```python
from build123d import *

# Parameters (mm, degrees)
SKETCH1_W           = 180
SKETCH1_H           = 87
BOSS_EXTRUDE1_DEPTH = 2
SKETCH6_W           = 2
SKETCH6_H           = 87
BOSS_EXTRUDE5_DEPTH = 5
SKETCH7_R           = 37.5
CUT_EXTRUDE2_DEPTH  = 5
SKETCH8_W           = 87
SKETCH8_H           = 87
SKETCH8_W_2         = 81
SKETCH8_H_2         = 81
BOSS_EXTRUDE6_DEPTH = 5
SKETCH9_W           = 150
SKETCH9_H           = 3
BOSS_EXTRUDE7_DEPTH = 5
SKETCH10_W          = 2
SKETCH10_H          = 87
CUT_EXTRUDE3_DEPTH  = 5
SKETCH11_W          = 2
SKETCH11_H          = 81
BOSS_EXTRUDE8_DEPTH = 5
SKETCH12_R          = 7.5
CUT_EXTRUDE4_DEPTH  = 5


with BuildPart() as part:
    # Sketch1 → Boss-Extrude1 (new body)
    with BuildSketch(Plane(origin=(0, 0, 0), x_dir=(1, 0, 0), z_dir=(0, 1, 0))):
        with Locations((31.597011279, 2.798063398)):
            Rectangle(SKETCH1_W, SKETCH1_H)
    extrude(amount=BOSS_EXTRUDE1_DEPTH)

    # Sketch6 → Boss-Extrude5 (add)
    with BuildSketch(Plane(origin=(0, 0, 0), x_dir=(-1, 0, 0), z_dir=(0, -1, 0))):
        with Locations((44.402988721, 2.798063398)):
            Rectangle(SKETCH6_W, SKETCH6_H)
        with Locations((-107.597011279, 2.798063398)):
            Rectangle(SKETCH6_W, SKETCH6_H)
    extrude(amount=BOSS_EXTRUDE5_DEPTH)

    # Sketch7 → Cut-Extrude2 (cut)
    with BuildSketch(Plane(origin=(0, 0, 0), x_dir=(-1, 0, 0), z_dir=(0, -1, 0))):
        with Locations((-31.597011279, 2.798063398)):
            Circle(SKETCH7_R)
    extrude(amount=-CUT_EXTRUDE2_DEPTH, mode=Mode.SUBTRACT)

    # Sketch8 → Boss-Extrude6 (add)
    with BuildSketch(Plane(origin=(0, 0, 0), x_dir=(-1, 0, 0), z_dir=(0, -1, 0))):
        with Locations((-31.597011279, 2.798063398)):
            Rectangle(SKETCH8_W, SKETCH8_H)
        with Locations((-31.597011279, 2.798063398)):
            Rectangle(SKETCH8_W_2, SKETCH8_H_2, mode=Mode.SUBTRACT)
    extrude(amount=BOSS_EXTRUDE6_DEPTH)

    # Sketch9 → Boss-Extrude7 (add)
    with BuildSketch(Plane(origin=(0, 0, 0), x_dir=(-1, 0, 0), z_dir=(0, -1, 0))):
        with Locations((-31.597011279, 44.798063398)):
            Rectangle(SKETCH9_W, SKETCH9_H)
        with Locations((-31.597011279, -39.201936602)):
            Rectangle(SKETCH9_W, SKETCH9_H)
    extrude(amount=BOSS_EXTRUDE7_DEPTH)

    # Sketch10 → Cut-Extrude3 (cut)
    with BuildSketch(Plane(origin=(0, -5, 0), x_dir=(-1, 0, 0), z_dir=(0, -1, 0))):
        with Locations((-107.597011279, 2.798063398)):
            Rectangle(SKETCH10_W, SKETCH10_H)
        with Locations((44.402988721, 2.798063398)):
            Rectangle(SKETCH10_W, SKETCH10_H)
    extrude(amount=-CUT_EXTRUDE3_DEPTH, mode=Mode.SUBTRACT)

    # Sketch11 → Boss-Extrude8 (add)
    with BuildSketch(Plane(origin=(0, 0, 0), x_dir=(-1, 0, 0), z_dir=(0, -1, 0))):
        with Locations((42.402988721, 2.798063398)):
            Rectangle(SKETCH11_W, SKETCH11_H)
        with Locations((-105.597011279, 2.798063398)):
            Rectangle(SKETCH11_W, SKETCH11_H)
    extrude(amount=BOSS_EXTRUDE8_DEPTH)

    # Sketch12 → Cut-Extrude4 (cut)
    with BuildSketch(Plane(origin=(0, 0, 0), x_dir=(-1, 0, 0), z_dir=(0, -1, 0))):
        with Locations((26.652988721, 23.048063398)):
            Circle(SKETCH12_R)
    extrude(amount=-CUT_EXTRUDE4_DEPTH, mode=Mode.SUBTRACT)


solid = part.part
```
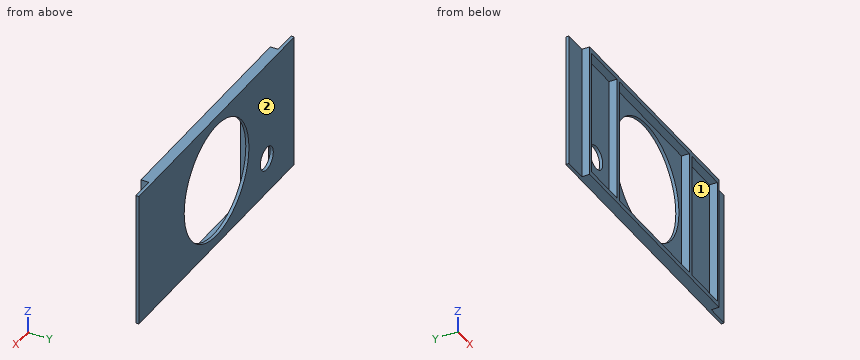
Geometry check sheet. Reference: the model listing, model coordinates, mm. Face numbers are marked on the shaded views. Give positions to 0.01 mm unless a question says otherwise; leave off trailing zeros. Order: outer loops, then holes, each group sorted by start corner. A loop starts at its lowest first (then second) coordinate and runs counter-clockwise, first axis right, second up. Notation, with made-up numbers: (29, 36) - (80, 36) arc R11 ccw to (80, 43) - close; hole circle Ø3 at (-3, 25.5). An arc over 180 degrees is marked (long way). Write item = value, one per line. Start each with the question number.
1) Scan lines: L1, parallel to X at y = -4.5, z = 25; L2, parallel to Z at x = 35, y = -4.5; L3, parallel to Y at x = 15, z = -37. Record each from-to range of solid material in increasing order.
2) Section check B-B (x = 35). Enter the section's corners in (y, z).
3) Section check C-C (z = 3). Enter the section's corners in (x, y), then the cut area to 3 significant figures.
4) Section check D-D (z = -26). Enter the section's corners in (x, y), then the cut area to 3 significant figures.
5) Gauge pin test, flat ends, axial feed: pin 1 Ø4 at (y, z) = (-2.5, 1) entering from -X; pin 2 Ø12 at (x, z) = (-54.5, -6) entering from -Y. Record the tip position at first contact, or that the pin passes through.
6) Section check A-A (y = -2.75). Enter the section's corners in (x, z), then the cut area to 3 significant figures.
7) Draft check along Z on the marked faces 1 and 2. Enter one of: released by +Z, released by -Z, zero draft, split by the parting line, or undercut.
Geometry check:
q1.L1 = -43.4 to -41.4, -11.9 to -8.9, 72.1 to 75.1, 104.6 to 106.6
q1.L2 = -46.3 to -43.3, 37.7 to 40.7
q1.L3 = 0 to 2
q2.outline = (-5, -46.3) - (2, -46.3) - (2, -40.14) - (0, -40.14) - (0, -43.3) - (-5, -43.3) - close; (-5, 37.7) - (0, 37.7) - (0, 34.55) - (2, 34.55) - (2, 40.7) - (-5, 40.7) - close
q3.outline = (-58.4, 0) - (-43.4, 0) - (-43.4, -5) - (-41.4, -5) - (-41.4, 0) - (-11.9, 0) - (-11.9, -5) - (-8.9, -5) - (-8.9, 0) - (-5.45, 0) - (-5.45, 2) - (-58.4, 2) - close; (68.65, 0) - (72.1, 0) - (72.1, -5) - (75.1, -5) - (75.1, 0) - (104.6, 0) - (104.6, -5) - (106.6, -5) - (106.6, 0) - (121.6, 0) - (121.6, 2) - (68.65, 2) - close
q3.area = 262 mm2
q4.outline = (-58.4, 0) - (-43.4, 0) - (-43.4, -5) - (-41.4, -5) - (-41.4, 0) - (-33.55, 0) - (-33.55, 2) - (-58.4, 2) - close; (-19.76, 0) - (-11.9, 0) - (-11.9, -5) - (-8.9, -5) - (-8.9, 0) - (2.14, 0) - (2.14, 2) - (-19.76, 2) - close; (61.06, 0) - (72.1, 0) - (72.1, -5) - (75.1, -5) - (75.1, 0) - (104.6, 0) - (104.6, -5) - (106.6, -5) - (106.6, 0) - (121.6, 0) - (121.6, 2) - (61.06, 2) - close
q4.area = 265 mm2
q5.pin_1 = -43.4
q5.pin_2 = 0
q6.outline = (-43.4, -46.3) - (106.6, -46.3) - (106.6, 40.7) - (-43.4, 40.7) - close; hole (-41.4, -43.3) - (-11.9, -43.3) - (-11.9, 37.7) - (-41.4, 37.7) - close; hole (-8.9, -43.3) - (72.1, -43.3) - (72.1, 37.7) - (-8.9, 37.7) - close; hole (75.1, -43.3) - (104.6, -43.3) - (104.6, 37.7) - (75.1, 37.7) - close
q6.area = 1,710 mm2
q7.face_1 = undercut
q7.face_2 = zero draft
